Build history of the part. All positions in model axes, mm. A direction names the side the tool comes from. Give positions to 0.01 mm unless a question says otherwise; leave off trailing zeros. Order: outer loops, then holes, each group sorted by start corner. A loop starts at its lowest first (then second) coordinate and runs counter-clockwise, first axis right, second up. Notation, with made-up numbers: (80, -29.5) - (90, -29.5) arc R26 cw to (90, -12.5) - close; hole circle Ø3 at (2.25, 79.5). An arc over 180 degrees is marked (long way). Use a Markdown table: item, result. Add a question column.
(1) Wall check: line 1 (Z direction, x = -51, y = -20); line 2 (Y direction, x = -53, z = 1); line 3 (X direction, y = -133, z = 122). Give the ranges that are in metal, low to high.
(2) Flat gauge pins, fed straight in: pin 1 (14.5 mm diameter, centred on y = -52.36, z = -23.51, fed in from +X); pin 2 (6 mm diameter, centred on x = -75, y = -106.5, fed in from +Z); pin 3 (6 mm diameter, centred on y = -152.5, z = 32.5, fed in from +X); pin 4 (8 mm diameter, centred on x = -65.5, y = -161.5, fed in from -Z). Where does each tip first touch, or does it go through?
(3) Mould opens along Y. For faces 1 (the face through (-4.93, -45.688, -19.098)), 2 (the face through (-30.28, 63.137, 34.471)), 3 (the face through (0, -37, 17)) say: +Y half, -Y half, draft (parallel to the pull), parting line (faces both ways), or undercut.
(4) Slice it at D-D (y = 100.5). Write the cut outline in (x, z), then the cut area to 3 significant figures.
(5) Slice it at C-C (x = -56). Write the cut outline in (y, z), then the cut area to 3 significant figures.
(6) Slice it at B-B (z = 0). Write the cut outline in (x, y), then the cut area to 3 significant figures.
(7) Which spindle directions (+Z, -Z, +X, -X, +Y, -Y) get a long thin tool onto all of the face, cutting with end or side? Do faces 4 (the face through (-4.93, -10.44, 30.55)), 5 (the face through (-50, -57, -83)), 6 (the face through (-10, -3, 17)). Say none if no direction does.
(8) Slice it at A-A (y = -20). Write the cut outline in (x, z).
from build123d import *

# Parameters (mm, degrees)
SCHIZZO3_R                  = 8
TAGLIO_ESTRUSIONE1_DEPTH    = 282.879406839
RIPETIZIONECIRCOLARE1_COUNT = 5
SMUSSO1_SIZE                = 10


with BuildPart() as part:
    # Schizzo2 → Rivoluzione1 (revolve)
    with BuildSketch(Plane.XY):
        Polygon((0, 0), (0, 70), (-50, 70), (-50, 160), (-84, 160), (-84, 60), (-10, 60), (-10, 0), align=None)
    revolve(axis=Axis((50, -20, 0), (-1, 0, 0)))

    # Schizzo3 → Taglio-Estrusione1 (cut, through all)
    with BuildSketch(Plane(origin=(0, 0, 0), x_dir=(0, 0, -1), z_dir=(1, 0, 0))):
        with Locations(Location((0, 20, 0), (0, 0, 90))):
            Circle(SCHIZZO3_R)
    taglio_estrusione1 = extrude(amount=-TAGLIO_ESTRUSIONE1_DEPTH, mode=Mode.SUBTRACT)

    # RipetizioneCircolare1: Taglio-Estrusione1 ×5 about axis
    ripetizionecircolare1_axis = Axis((0, -20, 0), (1, 0, 0))
    for i in range(1, RIPETIZIONECIRCOLARE1_COUNT):
        add(taglio_estrusione1.rotate(ripetizionecircolare1_axis, i * 360 / RIPETIZIONECIRCOLARE1_COUNT), mode=Mode.SUBTRACT)

    # Smusso1
    smusso1_edges = [part.edges().sort_by_distance(p)[0] for p in [
        (0, -110, 0),
    ]]
    chamfer(smusso1_edges, length=SMUSSO1_SIZE)


solid = part.part
Solution:
| question | item | result |
|---|---|---|
| 1 | line 1 | -180 to -80, 80 to 180 |
| 1 | line 2 | -200 to -99.99, 59.99 to 160 |
| 1 | line 3 | -84 to -50 |
| 2 | pin 1 | through |
| 2 | pin 2 | z = 159.46 |
| 2 | pin 3 | x = -50 |
| 2 | pin 4 | z = -116.16 |
| 3 | face 1 | undercut |
| 3 | face 2 | parting line |
| 3 | face 3 | draft |
| 4 | outline | (-84, -133.72) - (-50, -133.72) - (-50, 133.72) - (-84, 133.72) - close |
| 4 | area | 9,090 mm2 |
| 5 | outline | circle Ø360 at (-20, 0); hole circle Ø160 at (-20, 0) |
| 5 | area | 81,700 mm2 |
| 6 | outline | (-84, -200) - (-50, -200) - (-50, -110) - (-10, -110) - (0, -100) - (0, -40) - (-10, -40) - (-10, -100) - (-84, -100) - close; (-84, 60) - (-10, 60) - (-10, 28) - (0, 28) - (0, 60) - (-10, 70) - (-50, 70) - (-50, 160) - (-84, 160) - close; (-10, 0) - (0, 0) - (0, 12) - (-10, 12) - close |
| 6 | area | 8,740 mm2 |
| 7 | face 4 | +X, -X |
| 7 | face 5 | +X |
| 7 | face 6 | -X |
| 8 | outline | (-84, -180) - (-50, -180) - (-50, -90) - (-10, -90) - (0, -80) - (0, -20) - (-10, -20) - (-10, -80) - (-84, -80) - close; (-84, 80) - (-10, 80) - (-10, 20) - (0, 20) - (0, 80) - (-10, 90) - (-50, 90) - (-50, 180) - (-84, 180) - close |
